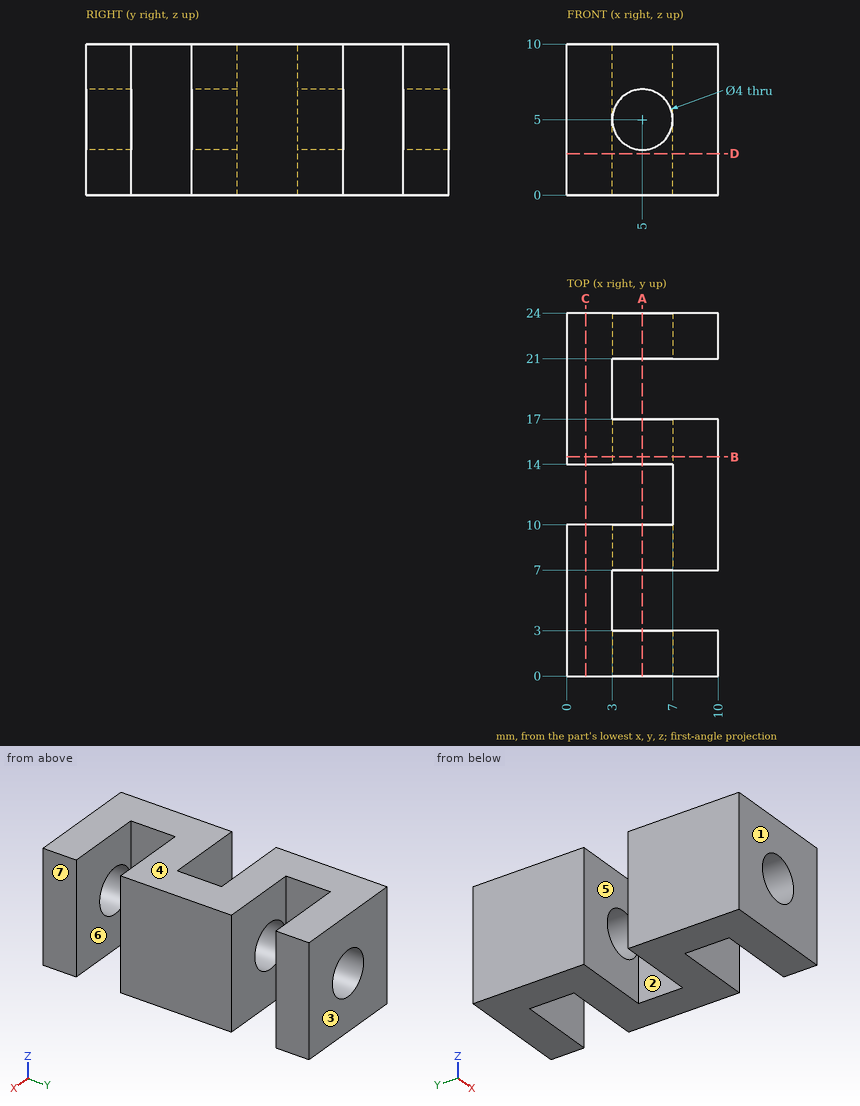
Here's the drawing with two shaded views (mm, measured from the low corner). I have some questions. A direction names the side the tool comes from. Coordinates: 2 decimals unless noted, no trailing zeros. Write each loop counter-clockwise with the first axis right and the second up, starting at its lowest first coordinate (ties: lowest second). Pieces come first, ordered by that corner, then holes. Notation, with made-up numbers: (33.25, 58) -> (61.25, 58) arc R10 ccw to (61.25, 64) -> close; hole circle Ø11 at (5.5, 30). An arc over 180 degrees is marked (long way). Write item = value, one per line. Start each with the question number.
(1) Will this pin go through, and if not, where does the flat tip stop? pin 1 (1.2 mm diameter, centred on y = 5.5, z = 7.5, fed in from +X).
(2) I need wall thicknesses on line 1 (Y direction, x = 6.75, z = 8.25); line 2 (Y direction, x = 7.5, z = 6); line 3 (Z direction, x = 5, y = 8.55). Which ranges of each line are inside material? Lowest first, please. Write a range as [from, to].
(3) I want a section at A-A (x = 5). Give the number of separate pieces and of enclosed holes in the cut face, plus the area to 3 significant figures.
(4) We'd pull the mould along Y, two halves only. Please class the marked faces 1, 2, 3 and 4: released by +Y, released by -Y, zero draft, split by the parting line, or undercut.
(5) I want a section at D-D (z = 2.75). Please give me the cut outline in (x, y), plus the area to 3 significant figures.
(6) I want a section at C-C (x = 1.25). Please give me the cut outline in (y, z).
(7) Which directions (+Z, -Z, +X, -X, +Y, -Y) give clear straight access to the entire face, cutting with the end or side of a thin tool? Please do the marked faces 5, 6 and 7.
(8) I want a section at B-B (y = 14.5). Please give me the cut outline in (x, z).
Result set:
q1.pin_1 = 3
q2.line_1 = [0, 3], [7, 10], [14, 17], [21, 24]
q2.line_2 = [0, 3], [7, 17], [21, 24]
q2.line_3 = [0, 3], [7, 10]
q3.separate_pieces = 8
q3.enclosed_holes = 0
q3.area = 72.0 mm2
q4.face_1 = released by -Y
q4.face_2 = undercut
q4.face_3 = released by +Y
q4.face_4 = zero draft
q5.outline = (0, 0) -> (10, 0) -> (10, 3) -> (3, 3) -> (3, 7) -> (10, 7) -> (10, 17) -> (3, 17) -> (3, 21) -> (10, 21) -> (10, 24) -> (0, 24) -> (0, 14) -> (7, 14) -> (7, 10) -> (0, 10) -> close
q5.area = 156 mm2
q6.outline = (0, 0) -> (10, 0) -> (10, 10) -> (0, 10) -> close; (14, 0) -> (24, 0) -> (24, 10) -> (14, 10) -> close
q7.face_5 = +Z, -Z, -X
q7.face_6 = +Z, -Z, +X
q7.face_7 = +Z, -Z, +X, +Y, -Y
q8.outline = (0, 0) -> (10, 0) -> (10, 10) -> (0, 10) -> close; hole circle Ø4 at (5, 5)
